Autodesk Inventor part; units mm, degrees
ref_plane "YZ Plane" through (0, 0, 0) normal (1, 0, 0) x (0, 1, 0)
ref_plane "XZ Plane" through (0, 0, 0) normal (0, 1, 0) x (-1, 0, 0)
ref_plane "XY Plane" through (0, 0, 0) normal (0, 0, 1) x (1, 0, 0)
sketch "Sketch1" plane through (0, 0, 0) normal (0, 1, 0) x (-1, 0, 0)
  line L0 (0.2032, -0.381) -> (-0.2032, -0.381)
  line L1 (-0.2032, -0.381) -> (-0.2032, 0.381)
  line L2 (-0.2032, 0.381) -> (0.2032, 0.381)
  line L3 (0.2032, 0.381) -> (0.2032, -0.381)
  line L4 (0.2032, -0.381) -> (-0.2032, 0.381) construction
  line L5 (-0.2032, -0.381) -> (0.2032, 0.381) construction
  point P0 (0, 0)
  dimension "d0" = 0.4064
  dimension "d1" = 0.762
extrude "Extrusion1" add sketch "Sketch1" along normal blind 15.4
chamfer "Chamfer1" distance 0.1 angle 45 8 edges at (0.2032, 15.4, 0) (0, 15.4, -0.381) (0, 15.4, 0.381) (-0.2032, 15.4, 0) (0.2032, 0, 0) (0, 0, -0.381) (0, 0, 0.381) (-0.2032, 0, 0)
sketch "Sketch2" plane through (-0.2032, 0.1, 0.381) normal (0, 0, 1) x (1, 0, 0)
  line L0 (-1.0405, 10.84) -> (1.7368, 10.84)
  point P0 (0.2032, -0.1)
  dimension "d7" = 10.94
bend part "Bend Part1" radius 1 angle 90 line through (-1.2437, 10.94, 0.381) along (1, 0, 0) centre toward (0, 0, 1) moving side (0, 1, 0) both sides no
properties part number "PinRight2" material "Gold"
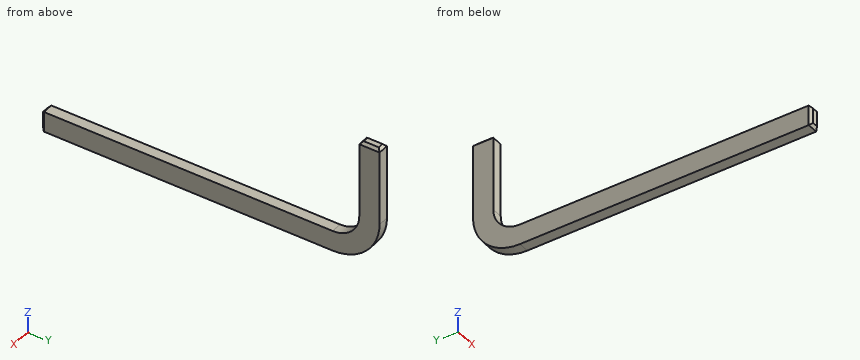
Geometry check sheet. Reference: the model listing, model coordinates, mm. Round coordinates to 2 decimals unless told otherwise and drop trailing zeros. Loops run counter-clockwise (first coordinate to the right, second up) from the corner with the lowest first, then second, coordinate; pieces in that order, holes last. Notation, with made-up numbers: (87.5, 36.25) -> (126.5, 36.25) arc R10 cw to (126.5, 51.25) -> close; hole circle Ø7 at (51, 17.25). An arc over 180 degrees is marked (long way). Answer as a JSON object with one key per item and string values. Group by question number.
Item 1: Cross-section at C-C, the plane y = 3.75. Record the cut outline in (x, z).
Item 2: Cross-section at B-B, the plane z = 3.1. Record the cut outline in (x, y).
Item 3: Thickness scan on line 1 along Y through (x, z) = (0, 3.5); line 2 along Z through (x, y) = (0.1, 8); line 3 along Y through (x, z) = (0, 0.75). Record the ranges inside material, lowest first.
Item 4: Cross-section at A-A, the plane x = 0. Record the cut outline in (y, z), plus the area to 3 significant figures.
Determined:
{
 "1": {"outline": "(-0.2, -0.38) -> (0.2, -0.38) -> (0.2, 0.38) -> (-0.2, 0.38) -> close"},
 "2": {"outline": "(-0.2, 11.94) -> (0.2, 11.94) -> (0.2, 12.7) -> (-0.2, 12.7) -> close"},
 "3": {"line 1": "y = 11.94 to 12.7", "line 2": "z = -0.38 to 0.38", "line 3": "y = 11.72 to 12.59"},
 "4": {"outline": "(0, -0.28) -> (0.1, -0.38) -> (10.94, -0.38) arc R1.76 ccw to (12.7, 1.38) -> (12.7, 4.17) -> (12.6, 4.27) -> (12.04, 4.27) -> (11.94, 4.17) -> (11.94, 1.38) arc R1 cw to (10.94, 0.38) -> (0.1, 0.38) -> (0, 0.28) -> close", "area": "12.2 mm²"}
}
